Can you work these out from the model? Positions are in its coordinate system, mm. A direction names the side the tool comes from. Coordinates: 2 decimals unless noted, no trailing zeros. Order: outer loops, then holes, each group sorted by start corner. A loop starts at its lowest first (then second) coordinate and runs counter-clockwise, first axis right, second up. Notation, with made-up numbers: (57, 11.25) -> (62, 11.25) arc R28 ccw to (62, 49.25) -> close; hole circle Ø10 at (4, 35). An arc over 180 degrees is marked (long way). Answer as a JSON object with one key per item and string values. Group by question number.
(1) For pin 1 (8 mm diameter, centred on y = 13.5, z = 12, fed in from -X); pin 2 (4 mm diameter, centred on x = 9, y = 4, fed in from +Z); pin 3 (4 mm diameter, centred on x = -3, z = -19.5, fed in from -Y), each with a flat end and sliding along its axis, tell me the tip position at first contact or that it passes through.
(2) Which directions (+Z, -Z, +X, -X, +Y, -Y) give clear straight access to the entire face, cutting with the end or side of a thin tool? Please do faces 1 (the cylindrical face through (7.395, -6.278, 19.935)), 2 (the cylindrical face through (14.45, -6.48, 20.58)), 3 (the cylindrical face through (-2.528, 14.832, -19.343)), 4 (the flat face through (10, 7.6, -23.2)).
(3) If we mould it in two halves opening along Y, with no side actions, what happens to faces 5 (the cylindrical face through (2.605, 15.821, -20.633)), 6 (the flat face through (-5, 10, -23)), 7 (the flat face through (13.9, 7, -21)), 8 (the flat face through (0, -20.4, 5.6))? For each: pulls with the +Y half, pulls with the -Y half, needs draft (parallel to the pull), parting line crosses it, or undercut.
(4) I want a section at A-A, the plane x = 6.5. List the corners of the cut face in (y, z) for me.
(5) I need wall thicknesses on line 1 (Y direction, x = 14.45, z = 0) (3 decimals); line 2 (Y direction, x = -0.15, z = 0) (3 decimals); line 3 (Y direction, x = 5.25, z = 0.5). Which ranges of each line are inside material? Lowest first, please.
from build123d import *

# Parameters (mm, degrees)
SMUSSO1_SIZE = 0.5
RACCORDO1_R  = 0.3
SMUSSO2_SIZE = 0.5


with BuildPart() as part:
    # Schizzo1 → Rivoluzione1 (revolve)
    with BuildSketch(Plane.XY, mode=Mode.PRIVATE) as rivoluzione1_sk:
        Polygon((-5, 26), (10, 26), (10, 24.25), (11, 24.25), (11, 24.75), (15, 24.75), (15, 23.575), (13.9, 23.575), (13.9, 21.575), (15, 21.575), (15, 20.9), (0, 20.9), (0, 24.875), (-0.5, 24.875), (-0.5, 24.375), (-5, 24.375), align=None)
    revolve(rivoluzione1_sk.sketch.rotate(Axis((0, 0, 0), (1, 0, 0)), 90), axis=Axis((0, 0, 0), (1, 0, 0)))  # turned: the seam where the file's is

    # Smusso1
    smusso1_edges = [part.edges().sort_by_distance(p)[0] for p in [
        (-5, 0, -24.375),
    ]]
    chamfer(smusso1_edges, length=SMUSSO1_SIZE)

    # Raccordo1
    raccordo1_edges = [part.edges().sort_by_distance(p)[0] for p in [
        (13.9, 0, -23.575),
        (13.9, 0, -21.575),
        (15, 0, -21.575),
    ]]
    fillet(raccordo1_edges, radius=RACCORDO1_R)

    # Smusso2
    smusso2_edges = [part.edges().sort_by_distance(p)[0] for p in [
        (15, 0, -24.75),
    ]]
    chamfer(smusso2_edges, length=SMUSSO2_SIZE)


solid = part.part
Computed values:
{
 "1": {"pin 1": "stops at x = 0", "pin 2": "stops at z = 25.92", "pin 3": "stops at y = -19.23"},
 "2": {"face 1": "+X, -X", "face 2": "+X", "face 3": "-X", "face 4": "none"},
 "3": {"face 5": "parting line crosses it", "face 6": "needs draft", "face 7": "undercut", "face 8": "undercut"},
 "4": {"outline": "circle Ø52 at (0, 0); hole circle Ø41.8 at (0, 0)"},
 "5": {"line 1": "y = -24.75 to -23.575, -21.575 to -20.9, 20.9 to 21.575, 23.575 to 24.75", "line 2": "y = -26 to -24.875, 24.875 to 26", "line 3": "y = -26 to -20.89, 20.89 to 26"}
}
